The model under review builds one solid part; all positions refer to its coordinate system, in mm. Round coordinates to 2 decimals unless told otherwise and drop trailing zeros. Answer as a JSON object with one key per item and string values. Group by question number.
1) We need section A-A, the plane x = 18. Count the separate pieces of the cut face and the enclosed holes in it, then the cut area to 3 significant figures.
2) To check wall thickness, follow probe 1 along Y at (x, z) = (21.5, -6.35); probe 2 along Y at (x, z) = (25, -6.35); probe 3 along Y at (x, z) = (36, -8). State the ranges of each line that lie inside material, in increasing order. Write a range as [from, to].
3) Insertion check: pin 1 Ø3 at (y, z) = (-5371.5, -5) entering from +X; pin 2 Ø2 at (x, z) = (49, -4.5) entering from -Y. Each pin has a flat end and moves straight along its axis. Give the tip position at first contact, or say it passes through.
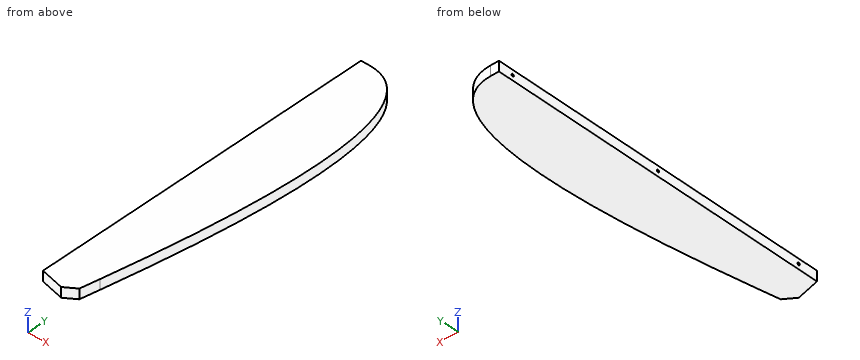
from build123d import *

# Parameters (mm, degrees)
BOSS_EXTRUDE1_DEPTH = 12.7
CHAMFER1_SIZE       = 12.7
CHAMFER1_SIZE2      = 12.14102868
HOLE1_D             = 3.175
HOLE1_DEPTH         = 50.8
HOLE1_CSINK_D       = 10.16
HOLE1_CSINK_ANGLE   = 82
HOLE1_TIP           = 0.953866233


with BuildPart() as part:
    # Sketch2 → Boss-Extrude1 (new body)
    with BuildSketch(Plane.XY):
        Polygon((12.7, -5480.416534997), (54.140557785, -5490.047588702), (136.525, -5040.331407449), (12.7, -5040.331407449), align=None)
    extrude(amount=-BOSS_EXTRUDE1_DEPTH)

    # Fillet1
    # a fillet whose section is not a circle: 406.4, 38.1 mm, written as the material it takes off along each edge
    with BuildSketch(Plane(origin=(136.525, -5040.331407449, 1050.356508865), x_dir=(-0.18019344316526936, -0.9836311925921447, 0), z_dir=(0, 0, -1))) as fillet1_piece_1:
        with BuildLine():
            Bezier((420.142603546, 0), (0, 0), (20.394886876, 111.330615302), weights=[1, 1, 1])
            Line((20.394886876, 111.330615302), (0, 0))
            Line((0, 0), (420.142603546, 0))
        make_face()
    extrude(amount=2113.413017729, mode=Mode.SUBTRACT)

    # Chamfer1
    chamfer1_edges = [part.edges().sort_by_distance(p)[0] for p in [
        (54.140557785, -5490.047588702, -6.35),
    ]]
    chamfer1_side = [part.faces().sort_by_distance(p)[0] for p in [
        (57.479307716, -5471.822183168, -6.35),
    ]]
    chamfer(chamfer1_edges, length=CHAMFER1_SIZE, length2=CHAMFER1_SIZE2, reference=chamfer1_side[0])

    # Hole1
    with Locations(Plane(origin=(-19.05, -5578.323279584, -94.73946), x_dir=(0, 0, 1), z_dir=(-1, 0, 0))):
        with Locations((218.563766336, 102.817509219), (218.563766336, 48.504773219), (202.68946, 123.306744588), (202.68946, 317.949308361), (202.68946, 518.941872135), (88.38946, 518.941872135), (88.38946, 317.949308361), (88.38946, 123.306744588), (104.263766336, 216.849631358), (104.263766336, 132.677202288), (104.263766336, 48.504773219), (-104.263766336, 48.504773219), (-104.263766336, 132.677202288), (-104.263766336, 216.849631358), (-88.38946, 123.306744588), (-88.38946, 317.949308361), (-88.38946, 518.941872135), (-202.68946, 518.941872135), (-202.68946, 317.949308361), (-202.68946, 123.306744588), (-218.563766336, 48.504773219), (-218.563766336, 102.817509219)):
            CounterSinkHole(HOLE1_D / 2, HOLE1_CSINK_D / 2, depth=HOLE1_DEPTH, counter_sink_angle=HOLE1_CSINK_ANGLE)
            with Locations((0, 0, -(HOLE1_DEPTH + HOLE1_TIP / 2))):  # 118° drill point
                Cone(0, HOLE1_D / 2, HOLE1_TIP, mode=Mode.SUBTRACT)


solid = part.part
Here are the results:
{
 "1": {"separate pieces": "1", "enclosed holes": "3", "area": "5,580 mm^2"},
 "2": {"probe 1": "y = [-5482.46, -5456.6], [-5453.43, -5261.96], [-5258.79, -5060.97], [-5057.79, -5040.33]", "probe 2": "y = [-5483.28, -5456.6], [-5453.43, -5261.96], [-5258.79, -5060.97], [-5057.79, -5040.35]", "probe 3": "y = [-5485.83, -5041.76]"},
 "3": {"pin 1": "stops at x = 74.84", "pin 2": "stops at y = -5483.37"}
}
